from build123d import *

# Parameters (mm, degrees)
F0_W     = 127
F0_H     = 76.2
F1_DEPTH = 14.224
F2_R     = 7.295041
F2_R_2   = 7.180955
F2_R_3   = 7.370116
F2_R_4   = 7.39498
F3_DEPTH = 27.94
F6_R     = 2.54
F7_SIZE  = 1.27


with BuildPart() as f1:
    # F0 (on Top) → F1 (new body)
    with BuildSketch(Plane.XY):
        Rectangle(F0_W, F0_H)
    extrude(amount=F1_DEPTH)

    # F2 (on Top) → F3 (cut)
    with BuildSketch(Plane.XY):
        with Locations((-52.690696, 27.844677)):
            Circle(F2_R)
        with Locations((51.833939, 27.844677)):
            Circle(F2_R_2)
        with Locations((52.6907, -28.701432)):
            Circle(F2_R_3)
        with Locations((-53.547453, -28.701432)):
            Circle(F2_R_4)
    extrude(amount=F3_DEPTH, mode=Mode.SUBTRACT)

    # F4 (on Front) → F5 (revolve)
    with BuildSketch(Plane.XZ):
        Polygon((12.7, 39.624), (0, 39.624), (0, 14.224), (12.7, 14.224), (12.776617, 20.498227), (5.493246, 20.498227), (5.493246, 25.638863), (5.493246, 32.492936), (12.7, 32.492936), align=None)
    revolve(axis=Axis((0, 0, 26.924), (0, 0, -1)))

    # F6
    f6_edges = [f1.edges().sort_by_distance(p)[0] for p in [
        (-12.7, 0, 39.624),
        (-12.7, 0, 14.224),
    ]]
    fillet(f6_edges, radius=F6_R)

    # F7
    f7_edges = [f1.edges().sort_by_distance(p)[0] for p in [
        (0, -38.1, 14.224),
        (63.5, 0, 14.224),
        (0, 38.1, 14.224),
        (-63.5, 0, 14.224),
    ]]
    chamfer(f7_edges, length=F7_SIZE)


solid = f1.part
Here's how the part is built. I have some questions about the finished solid (model axes, mm). A direction names the side the tool comes from. Round coordinates to 2 decimals unless told otherwise and drop trailing zeros. Order: outer loops, then holes, each group sorted by start corner. A loop starts at its lowest first (then second) coordinate and runs counter-clockwise, first axis right, second up. Notation, with made-up numbers: M 58.25,87.5 L 105.25,87.5 A27 ccw 105.25,124.5 Z; hole C 32,-13 d6. An arc over 180 degrees is marked long. Return JSON: item names as keys, results as strings. Group by question number.
1. If we section it at D-D on x = 22: List the corners of the cut face in (y, z) for me.
2. If we section it at C-C on z = 7: List the corners of the cut face in (x, y) for me, then the cut area to 3 significant figures.
3. On a 3-axis mill with a long thin cutter (end or side, diameter ignored), from which of +Z, -Z, +X, -X, +Y, -Y can I reach the whole of each face in a straight line? I mean faces 4 (the face through (-4.36, 3.34, 26.58)), 5 (the face through (-45.733, 30.036, 7.012)), 6 (the face through (-15, 9, 14.224)). Say none if no direction works.
4. I'm going to push flat-ended pins straight in: pin 1 Ø10 at (x, y) = (-10.5, 17.5) entering from +Z; pin 2 Ø6 at (y, z) = (8.5, 22) entering from +X; pin 3 Ø3 at (y, z) = (-15.5, 16) entering from -X. Where does each tip first touch, or does it pass through?
5. If we section it at B-B on x = 53: List the corners of the cut face in (y, z) for me.
6. If we mould it in two halves opening along X, with no side actions, what happens to faces 1 (the face through (46.541, 32.698, 7.012)), 2 (the face through (-2.765, 12.451, 18.673)), 3 (the face through (-5, 3, 32.493))? For each: pulls with the +X half, pulls with the -X half, needs draft (parallel to the pull), parting line crosses it, or undercut.
7. Please list where these lines run through material, in increasing order: probe 1 along Z at (x, y) = (-42, 28.5); probe 2 along X at (y, z) = (23.5, 6); probe 3 along X at (y, z) = (-11.5, 19).
8. If we section it at A-A on y = 24.5: List the corners of the cut face in (x, z) for me, then the cut area to 3 significant figures.
Reply:
{
 "1": {"outline": "M -38.1,0 L 38.1,0 L 38.1,12.95 L 36.83,14.22 L -36.83,14.22 L -38.1,12.95 Z"},
 "2": {"outline": "M -63.5,-38.1 L 63.5,-38.1 L 63.5,38.1 L -63.5,38.1 Z; hole C -53.55,-28.7 d14.79; hole C -52.69,27.84 d14.59; hole C 51.83,27.84 d14.36; hole C 52.69,-28.7 d14.74", "area": "9,010 mm^2"},
 "3": {"face 4": "none", "face 5": "+Z, -Z", "face 6": "+Z"},
 "4": {"pin 1": "z = 14.22", "pin 2": "x = 11.33", "pin 3": "through"},
 "5": {"outline": "M -38.1,0 L -36.07,0 L -36.07,14.22 L -36.83,14.22 L -38.1,12.95 Z; M -21.34,0 L 20.76,0 L 20.76,14.22 L -21.34,14.22 Z; M 34.93,0 L 38.1,0 L 38.1,12.95 L 36.83,14.22 L 34.93,14.22 Z"},
 "6": {"face 1": "undercut", "face 2": "parting line crosses it", "face 3": "needs draft"},
 "7": {"probe 1": "0 to 14.22", "probe 2": "-63.5 to -58.55, -46.83 to 46.12, 57.55 to 63.5", "probe 3": "-5.52 to 5.52"},
 "8": {"outline": "M -63.5,0 L -59.17,0 L -59.17,14.22 L -62.23,14.22 L -63.5,12.95 Z; M -46.21,0 L 45.48,0 L 45.48,14.22 L -46.21,14.22 Z; M 58.19,0 L 63.5,0 L 63.5,12.95 L 62.23,14.22 L 58.19,14.22 Z", "area": "1,440 mm^2"}
}
